from build123d import *

# Parameters (mm, degrees)
BOSS_EXTRUDE5_DEPTH  = 90
SKETCH11_3_R         = 55
BOSS_EXTRUDE6_DEPTH  = 115
SKETCH11_4_R         = 72
BOSS_EXTRUDE7_DEPTH  = 105
BOSS_EXTRUDE8_DEPTH  = 15
SKETCH17_R           = 45
BOSS_EXTRUDE9_DEPTH  = 80
SKETCH18_R           = 52
BOSS_EXTRUDE10_DEPTH = 5


with BuildPart() as part:
    # Sketch11 → Boss-Extrude5 (new body)
    with BuildSketch(Plane.XY):
        with BuildLine():
            ThreePointArc((-45, 56.204981986), (0, 72), (45, 56.204981986))
            Line((45, 56.204981986), (45, 350.377223398))
            ThreePointArc((45, 350.377223398), (0, 327), (-45, 350.377223398))
            Line((-45, 350.377223398), (-45, 56.204981986))
        make_face()
    extrude(amount=BOSS_EXTRUDE5_DEPTH)

    # Sketch11_3 → Boss-Extrude6 (add)
    with BuildSketch(Plane.XY):
        with Locations((0, 382)):
            Circle(SKETCH11_3_R)
    extrude(amount=BOSS_EXTRUDE6_DEPTH)

    # Sketch11_4 → Boss-Extrude7 (add)
    with BuildSketch(Plane.XY):
        Circle(SKETCH11_4_R)
    extrude(amount=BOSS_EXTRUDE7_DEPTH)

    # Sketch13 → Boss-Extrude8 (add)
    with BuildSketch(Plane.XY.offset(90)):
        with BuildLine():
            Line((10, 82), (10, 71.30217388))
            Line((10, 71.30217388), (-10, 71.30217388))
            Line((-10, 71.30217388), (-10, 82))
            ThreePointArc((-10, 82), (0, 92), (10, 82))
        make_face()
    extrude(amount=BOSS_EXTRUDE8_DEPTH)

    # Sketch17 → Boss-Extrude9 (add)
    with BuildSketch(Plane.XY.offset(115)):
        with Locations((0, 382)):
            Circle(SKETCH17_R)
    extrude(amount=BOSS_EXTRUDE9_DEPTH)

    # Sketch18 → Boss-Extrude10 (add)
    with BuildSketch(Plane(origin=(0, 0, 0), x_dir=(-1, 0, 0), z_dir=(0, 0, -1))):
        with Locations((0, 382)):
            Circle(SKETCH18_R)
    extrude(amount=BOSS_EXTRUDE10_DEPTH)


solid = part.part
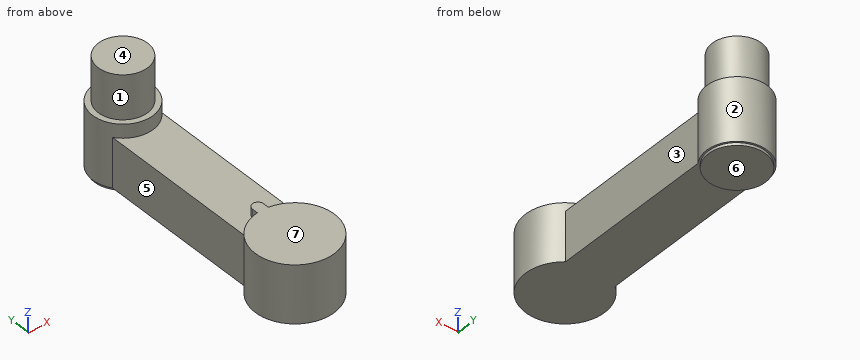
Can you work these out from the model? Positions are in its coordinate system, mm. Face numbers are marked on the shaded views. A direction names the side the tool comes from. Coordinates: 2 decimals unless noted, no trailing zeros. Write each loop counter-clockwise with the first axis right and the second up, starting at its lowest first coordinate (ties: lowest second). Pieces come first, ordered by that corner, then holes.
Q1. Please list where these lines run through material, in increasing order: L1, parallel to Z at x = -48, y = 6; L2, parallel to Z at x = 11.5, y = 138.5; L3, parallel to X at y = 176, z = 61.
Results found:
L1: z = 0 to 105
L2: z = 0 to 90
L3: x = -45 to 45
Q2. Imagine slicing it at B-B, the plane y = 382. List the corners of the cut face in (x, z) for me.
Results found:
outline: (-55, 0) - (-52, 0) - (-52, -5) - (52, -5) - (52, 0) - (55, 0) - (55, 115) - (45, 115) - (45, 195) - (-45, 195) - (-45, 115) - (-55, 115) - close
Q3. Imagine slicing it at C-C, the plane z = 175. List the corners of the cut face in (x, y) for me, plus the area to 3 significant figures.
Results found:
outline: circle Ø90 at (0, 382)
area: 6,360 mm2
Q4. Which directions (+Z, -Z, +X, -X, +Y, -Y) give clear straight access to the entire face, cutting with the end or side of a thin tool? Please do the marked faces 5, 6 and 7.
Results found:
face 5: +Z, -Z, -X
face 6: -Z, +X, -X, +Y, -Y
face 7: +Z, +X, -X, -Y
Q5. If we mould it in two halves opening along Y, with no side actions, what happens to the marked faces 1, 2, 3 and 4? For each: +Y half, -Y half, draft (parallel to the pull), parting line (faces both ways), or undercut.
Results found:
face 1: parting line
face 2: undercut
face 3: undercut
face 4: draft
Q6. Imagine slicing it at A-A, the plane x = 0. List the corners of the cut face in (y, z) for me.
Results found:
outline: (-72, 0) - (330, 0) - (330, -5) - (434, -5) - (434, 0) - (437, 0) - (437, 115) - (427, 115) - (427, 195) - (337, 195) - (337, 115) - (327, 115) - (327, 90) - (92, 90) - (92, 105) - (-72, 105) - close
Q7. For P1, Ø1.5, axis at y = 346, z = 46, coming from the -X side; P2, Ø12, axis at x = -26, y = 259, coming from the -Z side; P3, Ø8, axis at x = -26.5, z = 122.5, coming from the +Y side, each with a flat end and sliding along its axis, tell me the tip position at first contact or that it passes through.
Results found:
P1: stops at x = -45
P2: stops at z = 0
P3: stops at y = 420.97
Q8. Imagine slicing it at D-D, the plane y = 0. List the corners of the cut face in (x, z) for me, plus the area to 3 significant figures.
Results found:
outline: (-72, 0) - (72, 0) - (72, 105) - (-72, 105) - close
area: 15,100 mm2
